```python
from build123d import *

# Parameters (mm, degrees)
EXTRUDE_1_DEPTH     = 12
SKETCH_2_W          = 21
SKETCH_2_H          = 35.3
SKETCH_2_R          = 1.25
SKETCH_2_W_2        = 13
SKETCH_2_H_2        = 23.3
EXTRUDE_2_DEPTH     = 4
EXTRUDE_START       = -18
EXTRUDE_3_DEPTH     = 3
CHAMFER_1_SIZE      = 5
EXTRUDE_START_2     = -3
SKETCH_4_R          = 2
EXTRUDE_4_DEPTH     = 7
CUT_EXTRUDE_1_DEPTH = 12
SKETCH_6_R          = 1
CUT_EXTRUDE_2_DEPTH = 1.4
SKETCH_6_3_R        = 1
CUT_EXTRUDE_3_DEPTH = 4
SKETCH_7_R          = 2.925
EXTRUDE_5_DEPTH     = 4
SKETCH_8_R          = 1.5
CUT_EXTRUDE_4_DEPTH = 5
SKETCH_9_R          = 2.925
EXTRUDE_6_DEPTH     = 4
SKETCH_10_R         = 1.5
CUT_EXTRUDE_5_DEPTH = 5
SKETCH_11_R         = 2.5
EXTRUDE_7_DEPTH     = 0.4
SKETCH_12_R         = 2.5
EXTRUDE_8_DEPTH     = 0.4


with BuildPart() as part:
    # Sketch 1 → Extrude 1 (new body)
    with BuildSketch(Plane(origin=(0, 0, 0), x_dir=(1, 0, 0), z_dir=(0, 1, 0))):
        Polygon((0, 0), (20, 0), (20, 28.4), (0, 28.4), (0, 32.4), (24, 32.4), (41, 32.4), (41, -4), (37, -4), (37, 28.4), (24, 28.4), (24, -4), (0, -4), align=None)
    extrude(amount=EXTRUDE_1_DEPTH)

    # Sketch 2 → Extrude 2 (add)
    with BuildSketch(Plane.XY.offset(4)):
        with Locations((30.5, 11.65)):
            Rectangle(SKETCH_2_W, SKETCH_2_H)
        with Locations((27, 25.65)):
            Circle(SKETCH_2_R, mode=Mode.SUBTRACT)
        with Locations((27, -2.35)):
            Circle(SKETCH_2_R, mode=Mode.SUBTRACT)
        with Locations((34, -2.35)):
            Circle(SKETCH_2_R, mode=Mode.SUBTRACT)
        with Locations((34, 25.65)):
            Circle(SKETCH_2_R, mode=Mode.SUBTRACT)
        with Locations((30.5, 11.65)):
            Rectangle(SKETCH_2_W_2, SKETCH_2_H_2, mode=Mode.SUBTRACT)
    extrude(amount=-EXTRUDE_2_DEPTH)

    # Sketch 3 → Extrude 3 (add, symmetric)
    with BuildSketch(Plane(origin=(0, 0, -32.4), x_dir=(-1, 0, 0), z_dir=(0, 0, -1)).offset(EXTRUDE_START)):
        with BuildLine():
            Line((-41, 12), (-46, 12))
            Line((-46, 12), (-66.429561848, 9.473539494))
            ThreePointArc((-66.429561848, 9.473539494), (-69.5, 6), (-66.429561848, 2.526460506))
            Line((-66.429561848, 2.526460506), (-46, 0))
            Line((-46, 0), (-41, 0))
            Line((-41, 0), (-41, 12))
        make_face()
    extrude(amount=EXTRUDE_3_DEPTH, both=True)

    # Chamfer 1
    chamfer_1_edges = [part.edges().sort_by_distance(p)[0] for p in [
        (41, 6, -11.4),
        (41, 6, -17.4),
    ]]
    chamfer(chamfer_1_edges, length=CHAMFER_1_SIZE)

    # Sketch 4 → Extrude 4 (add, symmetric)
    with BuildSketch(Plane(origin=(0, 0, -17.4), x_dir=(-1, 0, 0), z_dir=(0, 0, -1)).offset(EXTRUDE_START_2)):
        with Locations((-66, 6)):
            Circle(SKETCH_4_R)
    extrude(amount=EXTRUDE_4_DEPTH, both=True)

    # Sketch 5 → Cut-Extrude 1 (cut)
    with BuildSketch(Plane(origin=(0, 0, -32.4), x_dir=(-1, 0, 0), z_dir=(0, 0, -1))):
        with BuildLine():
            Line((0, 10.15), (-5, 10.15))
            ThreePointArc((-5, 10.15), (-9.15, 6), (-5, 1.85))
            Line((-5, 1.85), (0, 1.85))
            Line((0, 1.85), (0, 10.15))
        make_face()
    extrude(amount=-CUT_EXTRUDE_1_DEPTH, mode=Mode.SUBTRACT)

    # Sketch 6 → Cut-Extrude 2 (cut)
    with BuildSketch(Plane(origin=(0, 0, -32.4), x_dir=(-1, 0, 0), z_dir=(0, 0, -1))):
        with BuildLine():
            ThreePointArc((-5.2075, 1.855190746), (-9.15, 6), (-5.2075, 10.144809254))
            Line((-5.2075, 10.144809254), (-18.175, 9.495622262))
            ThreePointArc((-18.175, 9.495622262), (-21.5, 6), (-18.175, 2.504377738))
            Line((-18.175, 2.504377738), (-5.2075, 1.855190746))
        make_face()
        with Locations((-15, 6)):
            Circle(SKETCH_6_R, mode=Mode.SUBTRACT)
        with Locations((-12, 6)):
            Circle(SKETCH_6_R, mode=Mode.SUBTRACT)
        with Locations((-18, 6)):
            Circle(SKETCH_6_R, mode=Mode.SUBTRACT)
    extrude(amount=-CUT_EXTRUDE_2_DEPTH, mode=Mode.SUBTRACT)

    # Sketch 6_3 → Cut-Extrude 3 (cut)
    with BuildSketch(Plane(origin=(0, 0, -32.4), x_dir=(-1, 0, 0), z_dir=(0, 0, -1))):
        with Locations((-18, 6)):
            Circle(SKETCH_6_3_R)
        with Locations((-15, 6)):
            Circle(SKETCH_6_3_R)
        with Locations((-12, 6)):
            Circle(SKETCH_6_3_R)
    extrude(amount=-CUT_EXTRUDE_3_DEPTH, mode=Mode.SUBTRACT)

    # Sketch 7 → Extrude 5 (add)
    with BuildSketch(Plane.XY.offset(4)):
        with Locations((5, 6)):
            Circle(SKETCH_7_R)
    extrude(amount=EXTRUDE_5_DEPTH)

    # Sketch 8 → Cut-Extrude 4 (cut)
    with BuildSketch(Plane.XY.offset(8)):
        with Locations((5, 6)):
            Circle(SKETCH_8_R)
    extrude(amount=-CUT_EXTRUDE_4_DEPTH, mode=Mode.SUBTRACT)

    # Sketch 9 → Extrude 6 (add)
    with BuildSketch(Plane(origin=(0, 0, -32.4), x_dir=(-1, 0, 0), z_dir=(0, 0, -1))):
        with Locations((-30.5, 6)):
            Circle(SKETCH_9_R)
    extrude(amount=EXTRUDE_6_DEPTH)

    # Sketch 10 → Cut-Extrude 5 (cut)
    with BuildSketch(Plane(origin=(0, 0, -36.4), x_dir=(-1, 0, 0), z_dir=(0, 0, -1))):
        with Locations((-30.5, 6)):
            Circle(SKETCH_10_R)
    extrude(amount=-CUT_EXTRUDE_5_DEPTH, mode=Mode.SUBTRACT)

    # Sketch 11 → Extrude 7 (add)
    with BuildSketch(Plane(origin=(0, 0, -17.4), x_dir=(-1, 0, 0), z_dir=(0, 0, -1))):
        with Locations((-66, 6)):
            Circle(SKETCH_11_R)
    extrude(amount=EXTRUDE_7_DEPTH)

    # Sketch 12 → Extrude 8 (add)
    with BuildSketch(Plane.XY.offset(-11.4)):
        with Locations((66, 6)):
            Circle(SKETCH_12_R)
    extrude(amount=EXTRUDE_8_DEPTH)


solid = part.part
```
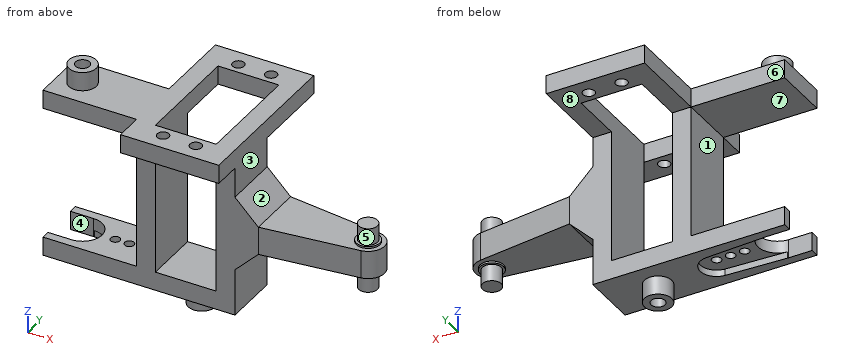
Here's how the part is built. I have some questions about the finished solid (model axes, mm). Face numbers are marked on the shaded views. A direction names the side the tool comes from. Round coordinates to 2 decimals unless told otherwise and drop trailing zeros. Write each loop counter-clockwise with the first axis right and the second up, starting at its lowest first coordinate (ties: lowest second). Pieces come first, ordered by that corner, then holes.
Q1. If we section it at C-C on x = 15: Write out the boundary of the cut face in (y, z), plus the area to 3 significant figures.
Q2. Will these pins go through, and if not, where does the flat tip stop? P1, Ø5, axis at x = 20.5, z = -8.5, coming from the +Y side; P2, Ø4, axis at x = 15, z = 3, coming from the -Y side; P3, Ø4, axis at x = 34, y = 25.65, coming from the -Z side.
Q3. Please list where these lines run through material, in increasing order: probe 1 along X at (y, z) = (7, -24); probe 2 along Y at (x, z) = (23, -27); probe 3 along Z at (x, y) = (37.5, 9).
Q4. If we section it at B-B on y = -2.35: Write out the boundary of the cut face in (x, z), plus the area to 3 significant figures.
Q5. If we section it at A-A on z = -27: Write out the boundary of the cut face in (x, y), plus the area to 3 significant figures.
Q6. Which directions (+Z, -Z, +X, -X, +Y, -Y) give clear straight access to the entire face, cutting with the end or side of a thin tool? Please do the marked faces 4, 5, 6, 7 and 8.
Q7. If we mould it in two halves opening along Z, with no side actions, what happens to the marked faces 1, 2 and 3? For each: +Z half, -Z half, draft (parallel to the pull), parting line (faces both ways), or undercut.
Q8. If we section it at D-D on y = 18: Write out the boundary of the cut face in (x, z).
Answer below:
1. outline: (0, -32.4) - (2.35, -32.4) - (2.35, -31) - (5, -31) - (5, -28.4) - (0, -28.4) - close; (0, 0) - (12, 0) - (12, 4) - (0, 4) - close; (7, -31) - (9.65, -31) - (9.65, -32.4) - (12, -32.4) - (12, -28.4) - (7, -28.4) - close
1. area: 80.6 mm2
2. P1: stops at y = 12
2. P2: stops at y = 0
2. P3: stops at z = 0
3. probe 1: x = 20 to 24, 37 to 41
3. probe 2: y = 0 to 12
3. probe 3: z = -32.4 to 4
4. outline: (20, 0) - (25.75, 0) - (25.75, 4) - (20, 4) - close; (28.25, 0) - (32.75, 0) - (32.75, 4) - (28.25, 4) - close; (35.25, 0) - (41, 0) - (41, 4) - (35.25, 4) - close
4. area: 64.0 mm2
5. outline: (20, 0) - (24, 0) - (24, 12) - (20, 12) - close; (37, 0) - (41, 0) - (41, 12) - (37, 12) - close
5. area: 96.0 mm2
6. face 4: -Z, -X
6. face 5: +Z
6. face 6: +Z, -Z, -X, +Y
6. face 7: -X, +Y, -Y
6. face 8: -Z, +X, -X, +Y
7. face 1: undercut
7. face 2: +Z half
7. face 3: draft
8. outline: (20, 0) - (24, 0) - (24, 4) - (20, 4) - close; (37, 0) - (41, 0) - (41, 4) - (37, 4) - close
